from build123d import *

# Parameters (mm, degrees)
SKETCH_W                = 55
SKETCH_H                = 55
PAD_DEPTH               = 380
POCKET_DEPTH            = 10
POLARPATTERN_COUNT      = 2
POLARPATTERN_ANGLE      = 90
BODY001_PLACEMENT_ANGLE = 90


with BuildPart() as part:
    # Sketch → Pad (new body)
    with BuildSketch(Plane.XY):
        Rectangle(SKETCH_W, SKETCH_H)
    extrude(amount=PAD_DEPTH)

    # Sketch001 (on DatumPlane) → Pocket (cut)
    with BuildSketch(Plane.YZ.offset(27.5)):
        Polygon((-10, 165), (-2.5, 165), (-2.5, 510), (2.5, 510), (2.5, 165), (10, 165), (10, 50), (-10, 50), align=None)
    pocket = extrude(amount=-POCKET_DEPTH, mode=Mode.SUBTRACT)

    # PolarPattern: Pocket ×2 about axis
    polarpattern_axis = Axis((0, 0, 0), (0, 0, 1))
    for i in range(1, POLARPATTERN_COUNT):
        add(pocket.rotate(polarpattern_axis, i * POLARPATTERN_ANGLE / (POLARPATTERN_COUNT - 1)), mode=Mode.SUBTRACT)


with BuildPart() as part_1:
    # Body placement: moved
    add(part.part.moved(Location((-10, 0, 0))))


with BuildPart() as part_2:
    # Clone placement: moved
    add(part_1.part.moved(Location((10, 0, 0))))


with BuildPart() as part_3:
    # Body001 placement: moved
    add(part_2.part.moved(Location((900, 0, 0))).rotate(Axis((900, 0, 0), (0, 0, 1)), BODY001_PLACEMENT_ANGLE))


solid = part_3.part
The model under review builds one solid part; all positions refer to its coordinate system, in mm. A direction names the side the tool comes from. Round coordinates to 2 decimals unless told otherwise and drop trailing zeros. Write each loop counter-clockwise with the first axis right and the second up, starting at its lowest first coordinate (ties: lowest second). Pieces come first, ordered by that corner, then holes. Notation, with made-up numbers: (82.25, 62) -> (113.25, 62) arc R13 ccw to (113.25, 84) -> close; hole circle Ø2 at (87.25, -31). An arc over 180 degrees is marked (long way). Answer as a JSON object with one key per item and string values.
1. We need section A-A on z = 150. State the section outline as (x, y) points.
Results found:
{"outline": "(872.5, -27.5) -> (927.5, -27.5) -> (927.5, 27.5) -> (910, 27.5) -> (910, 17.5) -> (890, 17.5) -> (890, 27.5) -> (872.5, 27.5) -> (872.5, 10) -> (882.5, 10) -> (882.5, -10) -> (872.5, -10) -> close"}
2. To check wall thickness, follow line 1 along Z through (x, y) = (878, -3.5); line 2 along X through (y, z) = (25.5, 307.5); line 3 along X through (y, z) = (18, 109). State the ranges of each line that lie inside material, in increasing order.
Results found:
{"line 1": "z = 0 to 50, 165 to 380", "line 2": "x = 872.5 to 897.5, 902.5 to 927.5", "line 3": "x = 872.5 to 890, 910 to 927.5"}
3. We need section C-C on z = 284.5. State the section outline as (x, y) points, and give its area (4 significant figures).
Results found:
{"outline": "(872.5, -27.5) -> (927.5, -27.5) -> (927.5, 27.5) -> (902.5, 27.5) -> (902.5, 17.5) -> (897.5, 17.5) -> (897.5, 27.5) -> (872.5, 27.5) -> (872.5, 2.5) -> (882.5, 2.5) -> (882.5, -2.5) -> (872.5, -2.5) -> close", "area": "2,925 mm^2"}
4. We need section B-B on x = 906. State the section outline as (y, z) points, and give its area (4 significant figures).
Results found:
{"outline": "(-27.5, 0) -> (27.5, 0) -> (27.5, 50) -> (17.5, 50) -> (17.5, 165) -> (27.5, 165) -> (27.5, 380) -> (-27.5, 380) -> close", "area": "19,750 mm^2"}
5. The part is to be moulded in two halves that separate along X. For faces 1 (the face through (877, 6, 165)), 2 (the face through (902.5, 23, 271)), 3 (the face through (872.5, -6, 187)), say which applies: pulls with the +X half, pulls with the -X half, needs draft (parallel to the pull), parting line crosses it, or undercut.
Results found:
{"face 1": "needs draft", "face 2": "undercut", "face 3": "pulls with the -X half"}
6. Clearance check with a flat-ended pin moving along its axis: pin 1 (1 mm diameter, centred on x = 904, z = 147.5, fed in from +Y). State where the tip first meets the part, or that it passes through.
Results found:
{"pin 1": "stops at y = 17.5"}
7. Machinability: for faces 4 (the face through (877, -6, 165)), 5 (the face through (906, 23, 165)), 6 (the face through (900, 0, 380)), 7 (the face through (877, 2.5, 271)), 8 (the face through (897.5, 23, 274)), which of the approach directions +Z, -Z, +X, -X, +Y, -Y give a long, thin tool a straight path to every point of the face, cutting with its end or side? Answer none if there is none.
Results found:
{"face 4": "-X", "face 5": "+Y", "face 6": "+Z, +X, -X, +Y, -Y", "face 7": "+Z, -X", "face 8": "+Z, +Y"}
